For this review, take the finished solid that the model builds, in its own axes (mm). Give positions to 0.01 mm unless a question says otherwise; leave off trailing zeros. Write each loop counter-clockwise with the first axis right and the second up, starting at its lowest first coordinate (ties: lowest second). Pieces come first, ordered by that corner, then holes.
1) We need section A-A on y = 114. Give the boundary of the cut face in (x, z).
2) We need section C-C on y = 143. Give the boundary of the cut face in (x, z), and give its area (3 significant figures).
3) We need section D-D on x = 7. Give the boundary of the cut face in (y, z), and give its area (3 significant figures).
4) Wall thickness on line 1 along X through (y, z) = (161.5, 17.7); line 2 along Y through (x, z) = (27.5, 17.3); line 3 along Y through (x, z) = (26.5, 18.1): over which ranges is each line inside the solid? List them lowest first.
5) We need section B-B on x = -22.5. Give the boundary of the cut face in (y, z), and give its area (3 significant figures).
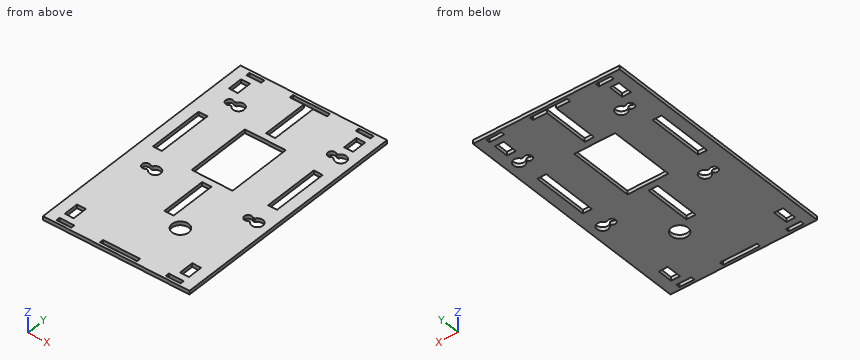
from build123d import *

# Parameters (mm, degrees)
SKETCH1_W              = 78.789320596
SKETCH1_H              = 130
PANEL_DEPTH            = 2
SUCKER_HOLES_REACH     = 206.318
FILLET1_R              = 0.5
SIDE_PLATE_SLOTS_REACH = 206.318
SKETCH3_W              = 22
SKETCH3_H              = 35
SKETCH3_W_2            = 5
SKETCH3_H_2            = 24.894660299
SKETCH3_W_3            = 8
SKETCH3_H_3            = 2
SKETCH3_W_4            = 4.8
SKETCH3_H_4            = 8
SKETCH3_H_5            = 30
SKETCH3_W_5            = 20
CUT_EXTRUDE3_REACH     = 206.318
SKETCH4_R              = 4.5


with BuildPart() as part:
    # Sketch1 → panel (new body)
    with BuildSketch(Plane.XY.offset(16.6)):
        with Locations((0, 135.474649456)):
            Rectangle(SKETCH1_W, SKETCH1_H)
    extrude(amount=PANEL_DEPTH)

    # Sketch2 → sucker holes (cut, up to next)
    with BuildSketch(Plane.XY.offset(18.6), mode=Mode.PRIVATE) as sucker_holes_sk1:
        with BuildLine():
            ThreePointArc((-26.177124344, 125.079989158), (-29.5, 123.579989158), (-26.177124344, 122.079989158))
            Line((-26.177124344, 122.079989158), (-25.098076211, 122.079989158))
            ThreePointArc((-25.098076211, 122.079989158), (-19.5, 123.579989158), (-25.098076211, 125.079989158))
            Line((-25.098076211, 125.079989158), (-26.177124344, 125.079989158))
        make_face()
    sucker_holes_tool1 = extrude(sucker_holes_sk1.sketch, amount=-SUCKER_HOLES_REACH, mode=Mode.PRIVATE) & part.part
    # Sketch2 → sucker holes (cut, up to next)
    with BuildSketch(Plane.XY.offset(18.6), mode=Mode.PRIVATE) as sucker_holes_sk2:
        with BuildLine():
            ThreePointArc((-26.177124344, 180.079989158), (-29.5, 178.579989158), (-26.177124344, 177.079989158))
            Line((-26.177124344, 177.079989158), (-25.098076211, 177.079989158))
            ThreePointArc((-25.098076211, 177.079989158), (-19.5, 178.579989158), (-25.098076211, 180.079989158))
            Line((-25.098076211, 180.079989158), (-26.177124344, 180.079989158))
        make_face()
    sucker_holes_tool2 = extrude(sucker_holes_sk2.sketch, amount=-SUCKER_HOLES_REACH, mode=Mode.PRIVATE) & part.part
    # Sketch2 → sucker holes (cut, up to next)
    with BuildSketch(Plane.XY.offset(18.6), mode=Mode.PRIVATE) as sucker_holes_sk3:
        with BuildLine():
            ThreePointArc((28.822875656, 180.079989158), (25.5, 178.579989158), (28.822875656, 177.079989158))
            Line((28.822875656, 177.079989158), (29.901923789, 177.079989158))
            ThreePointArc((29.901923789, 177.079989158), (35.5, 178.579989158), (29.901923789, 180.079989158))
            Line((29.901923789, 180.079989158), (28.822875656, 180.079989158))
        make_face()
    sucker_holes_tool3 = extrude(sucker_holes_sk3.sketch, amount=-SUCKER_HOLES_REACH, mode=Mode.PRIVATE) & part.part
    # Sketch2 → sucker holes (cut, up to next)
    with BuildSketch(Plane.XY.offset(18.6), mode=Mode.PRIVATE) as sucker_holes_sk4:
        with BuildLine():
            ThreePointArc((28.822875656, 125.079989158), (25.5, 123.579989158), (28.822875656, 122.079989158))
            Line((28.822875656, 122.079989158), (29.901923789, 122.079989158))
            ThreePointArc((29.901923789, 122.079989158), (35.5, 123.579989158), (29.901923789, 125.079989158))
            Line((29.901923789, 125.079989158), (28.822875656, 125.079989158))
        make_face()
    sucker_holes_tool4 = extrude(sucker_holes_sk4.sketch, amount=-SUCKER_HOLES_REACH, mode=Mode.PRIVATE) & part.part
    add(sucker_holes_tool1.solids().sort_by_distance((-24.075669, 123.579989, 18.6))[0], mode=Mode.SUBTRACT)
    add(sucker_holes_tool2.solids().sort_by_distance((-24.075669, 178.579989, 18.6))[0], mode=Mode.SUBTRACT)
    add(sucker_holes_tool3.solids().sort_by_distance((30.924331, 178.579989, 18.6))[0], mode=Mode.SUBTRACT)
    add(sucker_holes_tool4.solids().sort_by_distance((30.924331, 123.579989, 18.6))[0], mode=Mode.SUBTRACT)

    # Fillet1
    fillet1_edges = [part.edges().sort_by_distance(p)[0] for p in [
        (-26.177124344, 125.079989158, 17.6),
        (-25.098076211, 125.079989158, 17.6),
        (-25.098076211, 122.079989158, 17.6),
        (-26.177124344, 122.079989158, 17.6),
        (-25.098076211, 177.079989158, 17.6),
        (-26.177124344, 177.079989158, 17.6),
        (-26.177124344, 180.079989158, 17.6),
        (-25.098076211, 180.079989158, 17.6),
        (29.901923789, 177.079989158, 17.6),
        (28.822875656, 177.079989158, 17.6),
        (28.822875656, 180.079989158, 17.6),
        (29.901923789, 180.079989158, 17.6),
        (29.901923789, 122.079989158, 17.6),
        (28.822875656, 122.079989158, 17.6),
        (28.822875656, 125.079989158, 17.6),
        (29.901923789, 125.079989158, 17.6),
    ]]
    fillet(fillet1_edges, radius=FILLET1_R)

    # Sketch3 → side plate slots (cut, up to next)
    with BuildSketch(Plane.XY.offset(18.6), mode=Mode.PRIVATE) as side_plate_slots_sk1:
        with Locations((0, 151.079989158)):
            Rectangle(SKETCH3_W, SKETCH3_H)
    side_plate_slots_tool1 = extrude(side_plate_slots_sk1.sketch, amount=-SIDE_PLATE_SLOTS_REACH, mode=Mode.PRIVATE) & part.part
    # Sketch3 → side plate slots (cut, up to next)
    with BuildSketch(Plane.XY.offset(18.6), mode=Mode.PRIVATE) as side_plate_slots_sk2:
        Polygon((-2.5, 196.974649456), (-2.5, 172.079989158), (2.5, 172.079989158), (2.5, 196.974649456), (10, 196.974649456), (10, 198.974649456), (-10, 198.974649456), (-10, 196.974649456), align=None)
    side_plate_slots_tool2 = extrude(side_plate_slots_sk2.sketch, amount=-SIDE_PLATE_SLOTS_REACH, mode=Mode.PRIVATE) & part.part
    # Sketch3 → side plate slots (cut, up to next)
    with BuildSketch(Plane.XY.offset(18.6), mode=Mode.PRIVATE) as side_plate_slots_sk3:
        with Locations((0, 117.632659009)):
            Rectangle(SKETCH3_W_2, SKETCH3_H_2)
    side_plate_slots_tool3 = extrude(side_plate_slots_sk3.sketch, amount=-SIDE_PLATE_SLOTS_REACH, mode=Mode.PRIVATE) & part.part
    # Sketch3 → side plate slots (cut, up to next)
    with BuildSketch(Plane.XY.offset(18.6), mode=Mode.PRIVATE) as side_plate_slots_sk4:
        with Locations((-29.4, 72.974649456)):
            Rectangle(SKETCH3_W_3, SKETCH3_H_3)
    side_plate_slots_tool4 = extrude(side_plate_slots_sk4.sketch, amount=-SIDE_PLATE_SLOTS_REACH, mode=Mode.PRIVATE) & part.part
    # Sketch3 → side plate slots (cut, up to next)
    with BuildSketch(Plane.XY.offset(18.6), mode=Mode.PRIVATE) as side_plate_slots_sk5:
        with Locations((-29.4, 197.974649456)):
            Rectangle(SKETCH3_W_3, SKETCH3_H_3)
    side_plate_slots_tool5 = extrude(side_plate_slots_sk5.sketch, amount=-SIDE_PLATE_SLOTS_REACH, mode=Mode.PRIVATE) & part.part
    # Sketch3 → side plate slots (cut, up to next)
    with BuildSketch(Plane.XY.offset(18.6), mode=Mode.PRIVATE) as side_plate_slots_sk6:
        with Locations((29.4, 197.974649456)):
            Rectangle(SKETCH3_W_3, SKETCH3_H_3)
    side_plate_slots_tool6 = extrude(side_plate_slots_sk6.sketch, amount=-SIDE_PLATE_SLOTS_REACH, mode=Mode.PRIVATE) & part.part
    # Sketch3 → side plate slots (cut, up to next)
    with BuildSketch(Plane.XY.offset(18.6), mode=Mode.PRIVATE) as side_plate_slots_sk7:
        with Locations((-31, 189.474649456)):
            Rectangle(SKETCH3_W_4, SKETCH3_H_4)
    side_plate_slots_tool7 = extrude(side_plate_slots_sk7.sketch, amount=-SIDE_PLATE_SLOTS_REACH, mode=Mode.PRIVATE) & part.part
    # Sketch3 → side plate slots (cut, up to next)
    with BuildSketch(Plane.XY.offset(18.6), mode=Mode.PRIVATE) as side_plate_slots_sk8:
        with Locations((-31, 150.474649456)):
            Rectangle(SKETCH3_W_4, SKETCH3_H_5)
    side_plate_slots_tool8 = extrude(side_plate_slots_sk8.sketch, amount=-SIDE_PLATE_SLOTS_REACH, mode=Mode.PRIVATE) & part.part
    # Sketch3 → side plate slots (cut, up to next)
    with BuildSketch(Plane.XY.offset(18.6), mode=Mode.PRIVATE) as side_plate_slots_sk9:
        with Locations((-31, 81.474649456)):
            Rectangle(SKETCH3_W_4, SKETCH3_H_4)
    side_plate_slots_tool9 = extrude(side_plate_slots_sk9.sketch, amount=-SIDE_PLATE_SLOTS_REACH, mode=Mode.PRIVATE) & part.part
    # Sketch3 → side plate slots (cut, up to next)
    with BuildSketch(Plane.XY.offset(18.6), mode=Mode.PRIVATE) as side_plate_slots_sk10:
        with Locations((31, 81.474649456)):
            Rectangle(SKETCH3_W_4, SKETCH3_H_4)
    side_plate_slots_tool10 = extrude(side_plate_slots_sk10.sketch, amount=-SIDE_PLATE_SLOTS_REACH, mode=Mode.PRIVATE) & part.part
    # Sketch3 → side plate slots (cut, up to next)
    with BuildSketch(Plane.XY.offset(18.6), mode=Mode.PRIVATE) as side_plate_slots_sk11:
        with Locations((31, 150.474649456)):
            Rectangle(SKETCH3_W_4, SKETCH3_H_5)
    side_plate_slots_tool11 = extrude(side_plate_slots_sk11.sketch, amount=-SIDE_PLATE_SLOTS_REACH, mode=Mode.PRIVATE) & part.part
    # Sketch3 → side plate slots (cut, up to next)
    with BuildSketch(Plane.XY.offset(18.6), mode=Mode.PRIVATE) as side_plate_slots_sk12:
        with Locations((31, 189.474649456)):
            Rectangle(SKETCH3_W_4, SKETCH3_H_4)
    side_plate_slots_tool12 = extrude(side_plate_slots_sk12.sketch, amount=-SIDE_PLATE_SLOTS_REACH, mode=Mode.PRIVATE) & part.part
    # Sketch3 → side plate slots (cut, up to next)
    with BuildSketch(Plane.XY.offset(18.6), mode=Mode.PRIVATE) as side_plate_slots_sk13:
        with Locations((29.4, 72.974649456)):
            Rectangle(SKETCH3_W_3, SKETCH3_H_3)
    side_plate_slots_tool13 = extrude(side_plate_slots_sk13.sketch, amount=-SIDE_PLATE_SLOTS_REACH, mode=Mode.PRIVATE) & part.part
    # Sketch3 → side plate slots (cut, up to next)
    with BuildSketch(Plane.XY.offset(18.6), mode=Mode.PRIVATE) as side_plate_slots_sk14:
        with Locations((0, 72.974649456)):
            Rectangle(SKETCH3_W_5, SKETCH3_H_3)
    side_plate_slots_tool14 = extrude(side_plate_slots_sk14.sketch, amount=-SIDE_PLATE_SLOTS_REACH, mode=Mode.PRIVATE) & part.part
    add(side_plate_slots_tool1.solids().sort_by_distance((0, 151.079989, 18.6))[0], mode=Mode.SUBTRACT)
    add(side_plate_slots_tool2.solids().sort_by_distance((0, 187.797718, 18.6))[0], mode=Mode.SUBTRACT)
    add(side_plate_slots_tool3.solids().sort_by_distance((0, 117.632659, 18.6))[0], mode=Mode.SUBTRACT)
    add(side_plate_slots_tool4.solids().sort_by_distance((-29.4, 72.974649, 18.6))[0], mode=Mode.SUBTRACT)
    add(side_plate_slots_tool5.solids().sort_by_distance((-29.4, 197.974649, 18.6))[0], mode=Mode.SUBTRACT)
    add(side_plate_slots_tool6.solids().sort_by_distance((29.4, 197.974649, 18.6))[0], mode=Mode.SUBTRACT)
    add(side_plate_slots_tool7.solids().sort_by_distance((-31, 189.474649, 18.6))[0], mode=Mode.SUBTRACT)
    add(side_plate_slots_tool8.solids().sort_by_distance((-31, 150.474649, 18.6))[0], mode=Mode.SUBTRACT)
    add(side_plate_slots_tool9.solids().sort_by_distance((-31, 81.474649, 18.6))[0], mode=Mode.SUBTRACT)
    add(side_plate_slots_tool10.solids().sort_by_distance((31, 81.474649, 18.6))[0], mode=Mode.SUBTRACT)
    add(side_plate_slots_tool11.solids().sort_by_distance((31, 150.474649, 18.6))[0], mode=Mode.SUBTRACT)
    add(side_plate_slots_tool12.solids().sort_by_distance((31, 189.474649, 18.6))[0], mode=Mode.SUBTRACT)
    add(side_plate_slots_tool13.solids().sort_by_distance((29.4, 72.974649, 18.6))[0], mode=Mode.SUBTRACT)
    add(side_plate_slots_tool14.solids().sort_by_distance((0, 72.974649, 18.6))[0], mode=Mode.SUBTRACT)

    # Sketch4 → Cut-Extrude3 (cut, up to next)
    with BuildSketch(Plane.XY.offset(18.6), mode=Mode.PRIVATE) as cut_extrude3_sk1:
        with Locations((10, 100.474649456)):
            Circle(SKETCH4_R)
    cut_extrude3_tool1 = extrude(cut_extrude3_sk1.sketch, amount=-CUT_EXTRUDE3_REACH, mode=Mode.PRIVATE) & part.part
    add(cut_extrude3_tool1.solids().sort_by_distance((10, 100.474649, 18.6))[0], mode=Mode.SUBTRACT)


solid = part.part
Results list:
1. outline: (-39.39, 16.6) - (-2.5, 16.6) - (-2.5, 18.6) - (-39.39, 18.6) - close; (2.5, 16.6) - (39.39, 16.6) - (39.39, 18.6) - (2.5, 18.6) - close
2. outline: (-39.39, 16.6) - (-33.4, 16.6) - (-33.4, 18.6) - (-39.39, 18.6) - close; (-28.6, 16.6) - (-11, 16.6) - (-11, 18.6) - (-28.6, 18.6) - close; (11, 16.6) - (28.6, 16.6) - (28.6, 18.6) - (11, 18.6) - close; (33.4, 16.6) - (39.39, 16.6) - (39.39, 18.6) - (33.4, 18.6) - close
2. area: 94.4 mm2
3. outline: (70.47, 16.6) - (71.97, 16.6) - (71.97, 18.6) - (70.47, 18.6) - close; (73.97, 16.6) - (97.12, 16.6) - (97.12, 18.6) - (73.97, 18.6) - close; (103.83, 16.6) - (133.58, 16.6) - (133.58, 18.6) - (103.83, 18.6) - close; (168.58, 16.6) - (196.97, 16.6) - (196.97, 18.6) - (168.58, 18.6) - close; (198.97, 16.6) - (200.47, 16.6) - (200.47, 18.6) - (198.97, 18.6) - close
3. area: 169 mm2
4. line 1: x = -39.39 to -33.4, -28.6 to -11, 11 to 28.6, 33.4 to 39.39
4. line 2: y = 70.47 to 71.97, 73.97 to 121.58, 125.58 to 176.58, 180.58 to 196.97, 198.97 to 200.47
4. line 3: y = 70.47 to 71.97, 73.97 to 121.85, 125.31 to 176.85, 180.31 to 196.97, 198.97 to 200.47
5. outline: (70.47, 16.6) - (120.58, 16.6) - (120.58, 18.6) - (70.47, 18.6) - close; (126.58, 16.6) - (175.58, 16.6) - (175.58, 18.6) - (126.58, 18.6) - close; (181.58, 16.6) - (200.47, 16.6) - (200.47, 18.6) - (181.58, 18.6) - close
5. area: 236 mm2
